Here's how the part is built. I have some questions about the finished solid (model axes, mm). A direction names the side the tool comes from. Give positions to 0.01 mm unless a question says otherwise; leave off trailing zeros. Loops run counter-clockwise (first coordinate to the right, second up) from the corner with the lowest first, then second, coordinate; pieces in that order, holes last. Notation, with made-up numbers: (-34.5, -9.5) - (-2.5, -9.5) arc R8 cw to (-2.5, -4.5) - close; hole circle Ø5 at (-25, 53). An arc over 180 degrees is marked (long way). Put each result on its own line as item: value. Start each with the question number.
from build123d import *

# Parameters (mm, degrees)
SKIZZE1_W                             = 40
SKIZZE1_H                             = 110
AUFSATZ_LINEAR_AUSTRAGEN1_DEPTH       = 10
SKIZZE2_W                             = 40
SKIZZE2_H                             = 0.1
SCHNITT_LINEAR_AUSTRAGEN1_DEPTH       = 0.1
SKIZZE3_R                             = 11
SCHNITT_LINEAR_AUSTRAGEN2_DEPTH       = 11
SKIZZE5_R                             = 11
SCHNITT_LINEAR_AUSTRAGEN4_DEPTH       = 8
SKIZZE6_R                             = 10
SCHNITT_LINEAR_AUSTRAGEN5_DEPTH       = 8
FASE1_SIZE                            = 1
SKIZZE10_W                            = 40
SKIZZE10_H                            = 10
AUFSATZ_LINEAR_AUSTRAGEN2_DEPTH       = 9.7
SKIZZE11_R                            = 3
SCHNITT_LINEAR_AUSTRAGEN6_DEPTH       = 21
SKIZZE12_R                            = 4.5
SCHNITT_LINEAR_AUSTRAGEN11_DEPTH      = 13
SKIZZE15_R                            = 15.675658378
AUFSATZ_LINEAR_AUSTRAGEN3_DEPTH       = 2.5
SCHNITT_LINEAR_AUSTRAGEN13_DEPTH      = 3
SCHNITT_LINEAR_AUSTRAGEN13_DEPTH_BACK = 15
SKIZZE13_R                            = 10


with BuildPart() as part:
    # Skizze1 → Aufsatz-Linear austragen1 (new body)
    with BuildSketch(Plane.XY):
        with Locations((20, 55)):
            Rectangle(SKIZZE1_W, SKIZZE1_H)
    extrude(amount=AUFSATZ_LINEAR_AUSTRAGEN1_DEPTH)

    # Skizze2 → Schnitt-Linear austragen1 (cut)
    with BuildSketch(Plane(origin=(0, 0, 0), x_dir=(-1, 0, 0), z_dir=(0, 0, -1))):
        with Locations((-20, 10.55)):
            Rectangle(SKIZZE2_W, SKIZZE2_H)
    extrude(amount=-SCHNITT_LINEAR_AUSTRAGEN1_DEPTH, mode=Mode.SUBTRACT)

    # Skizze3 → Schnitt-Linear austragen2 (cut)
    with BuildSketch(Plane(origin=(0, 0, 0.1), x_dir=(-1, 0, 0), z_dir=(0, 0, -1))):
        with Locations((-20, 31.5)):
            Circle(SKIZZE3_R)
    extrude(amount=-SCHNITT_LINEAR_AUSTRAGEN2_DEPTH, mode=Mode.SUBTRACT)

    # Skizze5 → Schnitt-Linear austragen4 (cut)
    with BuildSketch(Plane.XY.offset(10)):
        with Locations((20.290455997, 96.8)):
            Circle(SKIZZE5_R)
    extrude(amount=-SCHNITT_LINEAR_AUSTRAGEN4_DEPTH, mode=Mode.SUBTRACT)

    # Skizze6 → Schnitt-Linear austragen5 (cut)
    with BuildSketch(Plane.XY.offset(2)):
        with Locations((20.290455997, 96.8)):
            Circle(SKIZZE6_R)
    extrude(amount=-SCHNITT_LINEAR_AUSTRAGEN5_DEPTH, mode=Mode.SUBTRACT)

    # Fase1
    fase1_edges = [part.edges().sort_by_distance(p)[0] for p in [
        (31, 31.5, 10),
        (9.290455997, 96.8, 10),
    ]]
    chamfer(fase1_edges, length=FASE1_SIZE)

    # Skizze10 → Aufsatz-Linear austragen2 (add)
    with BuildSketch(Plane.XY.offset(10)):
        with Locations((20, 5)):
            Rectangle(SKIZZE10_W, SKIZZE10_H)
    extrude(amount=AUFSATZ_LINEAR_AUSTRAGEN2_DEPTH)

    # Skizze11 → Schnitt-Linear austragen6 (cut)
    with BuildSketch(Plane(origin=(0, 0, 0), x_dir=(-1, 0, 0), z_dir=(0, 0, -1))):
        with Locations((-32.5, 5)):
            Circle(SKIZZE11_R)
        with Locations((-7.5, 5)):
            Circle(SKIZZE11_R)
    extrude(amount=-SCHNITT_LINEAR_AUSTRAGEN6_DEPTH, mode=Mode.SUBTRACT)

    # Skizze12 → Schnitt-Linear austragen11 (cut)
    with BuildSketch(Plane(origin=(0, 0, 0), x_dir=(-1, 0, 0), z_dir=(0, 0, -1))):
        with Locations((-32.5, 5)):
            Circle(SKIZZE12_R)
        with Locations((-7.5, 5)):
            Circle(SKIZZE12_R)
    extrude(amount=-SCHNITT_LINEAR_AUSTRAGEN11_DEPTH, mode=Mode.SUBTRACT)

    # Skizze15 → Aufsatz-Linear austragen3 (add)
    with BuildSketch(Plane.XY.offset(0.1)):
        with Locations((20, 31.5)):
            Circle(SKIZZE15_R)
    extrude(amount=AUFSATZ_LINEAR_AUSTRAGEN3_DEPTH)

    # Skizze13 → Schnitt-Linear austragen13 (cut, two sides: drawn at the far end of the back side and taken through both)
    with BuildSketch(Plane(origin=(0, 0, 0.1), x_dir=(-1, 0, 0), z_dir=(0, 0, -1)).offset(-SCHNITT_LINEAR_AUSTRAGEN13_DEPTH_BACK)):
        with Locations(Location((-20, 31.5, 0), (0, 0, 180))):
            Circle(SKIZZE13_R)
    extrude(amount=SCHNITT_LINEAR_AUSTRAGEN13_DEPTH + SCHNITT_LINEAR_AUSTRAGEN13_DEPTH_BACK, mode=Mode.SUBTRACT)


solid = part.part
1) I need wall thicknesses on line 1 (X direction, y = 96.5, z = 6.25); line 2 (Y direction, x = 32.5, z = 14.5); line 3 (Y direction, x = 12.5, z = 4.75). Which ranges of each line are inside material? Lowest first, please.
2) Thinking about a two-plate mould opening in X: for faces 6 (the flat face through (34, 2, 13)), 7 (the flat face through (40, 54, 5)), 8 (the flat face through (20, 61, 0)), which applies, pulls with the +X half, pulls with the -X half, needs draft (parallel to the pull), parting line crosses it, or undercut?
3) I'm going to push flat-ended pins straight in: P1, Ø8, axis at x = 19, y = 25.5, coming from the -Z side; P2, Ø3, axis at x = 29, y = 35, coming from the +Z side; P3, Ø24, axis at x = 17, y = 95.5, coming from the +Z side; P4, Ø17.5, axis at x = 20, y = 31.5, coming from the -Z side. Where does each tip first touch, or does it pass through?
4) Suppose I cut it at A-A on y = 96.8. Please give me the cut outline in (x, z), plus the area to 3 significant figures.
5) Suppose I cut it at D-D on z = 5.75. Please give me the cut outline in (x, y).
6) Which directions (+Z, -Z, +X, -X, +Y, -Y) give clear straight access to the entire face, cutting with the end or side of a thin tool? Please do faces 1 (the flat face through (20, 0, 10)), 2 (the cylindrical face through (28.34, 3.28, 6.41)), 3 (the flat face through (20, 61, 10)), 4 (the flat face through (23, 87, 2)), 5 (the cylindrical face through (35.5, 5.1, 16.3)).
7) Suppose I cut it at C-C on y = 5. Please give me the cut outline in (x, z).
8) Suppose I cut it at B-B on x = 6.5. Please give me the cut outline in (y, z), plus the area to 3 significant figures.
Ans:
1. line 1: x = 0 to 9.29, 31.29 to 40
1. line 2: y = 0 to 2, 8 to 10
1. line 3: y = 0 to 23.45, 39.55 to 89.03, 104.57 to 110
2. face 6: undercut
2. face 7: pulls with the +X half
2. face 8: needs draft
3. P1: stops at z = 0
3. P2: stops at z = 9.16
3. P3: stops at z = 10
3. P4: passes through
4. outline: (0, 0) - (10.29, 0) - (10.29, 2) - (9.29, 2) - (9.29, 9) - (8.29, 10) - (0, 10) - close; (30.29, 0) - (40, 0) - (40, 10) - (32.29, 10) - (31.29, 9) - (31.29, 2) - (30.29, 2) - close
4. area: 183 mm²
5. outline: (0, 0) - (40, 0) - (40, 110) - (0, 110) - close; hole circle Ø9 at (7.5, 5); hole circle Ø22 at (20, 31.5); hole circle Ø22 at (20.29, 96.8); hole circle Ø9 at (32.5, 5)
6. face 1: +Z, -Z, +X, -X, -Y
6. face 2: -Z
6. face 3: +Z, +X, -X, +Y
6. face 4: +Z
6. face 5: +Z, -Z
7. outline: (0, 0) - (3, 0) - (3, 13) - (4.5, 13) - (4.5, 19.7) - (0, 19.7) - close; (10.5, 13) - (12, 13) - (12, 0) - (28, 0) - (28, 13) - (29.5, 13) - (29.5, 19.7) - (10.5, 19.7) - close; (35.5, 13) - (37, 13) - (37, 0) - (40, 0) - (40, 19.7) - (35.5, 19.7) - close
8. outline: (0, 0) - (0.61, 0) - (0.61, 13) - (2.17, 13) - (2.17, 19.7) - (0, 19.7) - close; (7.83, 13) - (9.39, 13) - (9.39, 0) - (10.5, 0) - (10.5, 0.1) - (10.6, 0.1) - (10.6, 0) - (110, 0) - (110, 10) - (10, 10) - (10, 19.7) - (7.83, 19.7) - close
8. area: 1,050 mm²
